Here's how the part is built. I have some questions about the finished solid (model axes, mm). Coordinates: 2 decimals unless noted, no trailing zeros. Write each loop counter-clockwise with the first axis right and the second up, starting at its lowest first coordinate (ties: lowest second). Pieces come first, ordered by that corner, then holes. Notation, with made-up numbers: M -23.75,20 L 16.25,20 A22 cw 16.25,59 Z; hole C 86,61 d11. An arc over 180 degrees is marked long. Use one line per item in the form item = value. Start each with the question number.
1. I'm going to push flat-ended pins straight in: pin 1 Ø1.2 at (x, y) = (0, 25.5) entering from +Z; pin 2 Ø0.6 at (y, z) = (26.5, 1) entering from +X. Where does each tip first touch, or does it pass through?
2. I want a section at A-A, the plane x = 0. List the corners of the cut face in (y, z) for me, plus the area to 3 significant figures.
3. I want a section at B-B, the plane z = 1.2. List the corners of the cut face in (x, y) for me, plus the area to 3 significant figures.
4. I want a section at C-C, the plane y = 25.25. List the corners of the cut face in (x, z) for me, plus the area to 3 significant figures.
5. Please list where these lines run through material, in increasing order: line 1 along Y through (x, z) = (0, 1.35); line 2 along Y through (x, z) = (1.1, 1.25); line 3 along Y through (x, z) = (1.05, 1.9). Write a range as [from, to].
6. Thinking about a two-plate mould opening in X: for faces 1 (the face through (-0.108, -0.488, 0.986)), 2 (the face through (0, 24.5, 1)), 3 (the face through (0, 13, 0)), 4 (the face through (-1.254, 26.323, 0.986)), which applies, released by +X, released by -X, zero draft, split by the parting line, or undercut?
from build123d import *

# Parameters (mm, degrees)
SKETCH_1_R          = 0.5
EXTRUDE_1_DEPTH     = 2
CUT_EXTRUDE_1_DEPTH = 10


with BuildPart() as part:
    # 草图1 → 凸台-拉伸1 (new body)
    with BuildSketch(Plane.XY):
        with BuildLine():
            Line((-1.5, 25.5), (-1.5, 0))
            ThreePointArc((-1.5, 0), (0, -1.5), (1.5, 0))
            Line((1.5, 0), (1.5, 25.5))
            ThreePointArc((1.5, 25.5), (0, 27), (-1.5, 25.5))
        make_face()
        Circle(SKETCH_1_R, mode=Mode.SUBTRACT)
    extrude(amount=EXTRUDE_1_DEPTH)

    # 草图2 → 切除-拉伸1 (cut)
    with BuildSketch(Plane.XY.offset(2)):
        with BuildLine():
            Line((-0.5, 26.866025404), (-0.5, 26.366025404))
            ThreePointArc((-0.5, 26.366025404), (0, 24.5), (0.5, 26.366025404))
            Line((0.5, 26.366025404), (0.5, 26.866025404))
            Line((0.5, 26.866025404), (0.619656837, 26.866025404))
            ThreePointArc((0.619656837, 26.866025404), (0, 27), (-0.619656837, 26.866025404))
            Line((-0.619656837, 26.866025404), (-0.5, 26.866025404))
        make_face()
    extrude(amount=-CUT_EXTRUDE_1_DEPTH, mode=Mode.SUBTRACT)


solid = part.part
Answer list:
q1.pin_1 = through
q1.pin_2 = 1.33
q2.outline = M -1.5,0 L -0.5,0 L -0.5,2 L -1.5,2 Z; M 0.5,0 L 24.5,0 L 24.5,2 L 0.5,2 Z
q2.area = 50.0 mm²
q3.outline = M -1.5,0 A1.5 ccw 1.5,0 L 1.5,25.5 A1.5 ccw 0.62,26.87 L 0.5,26.87 L 0.5,26.37 A1 cw long -0.5,26.37 L -0.5,26.87 L -0.62,26.87 A1.5 ccw -1.5,25.5 Z; hole C 0,0 d1
q3.area = 79.1 mm²
q4.outline = M -1.5,0 L -0.97,0 L -0.97,2 L -1.5,2 Z; M 0.97,0 L 1.5,0 L 1.5,2 L 0.97,2 Z
q4.area = 2.13 mm²
q5.line_1 = [-1.5, -0.5], [0.5, 24.5]
q5.line_2 = [-1.02, 26.52]
q5.line_3 = [-1.07, 26.57]
q6.face_1 = undercut
q6.face_2 = undercut
q6.face_3 = zero draft
q6.face_4 = released by -X
